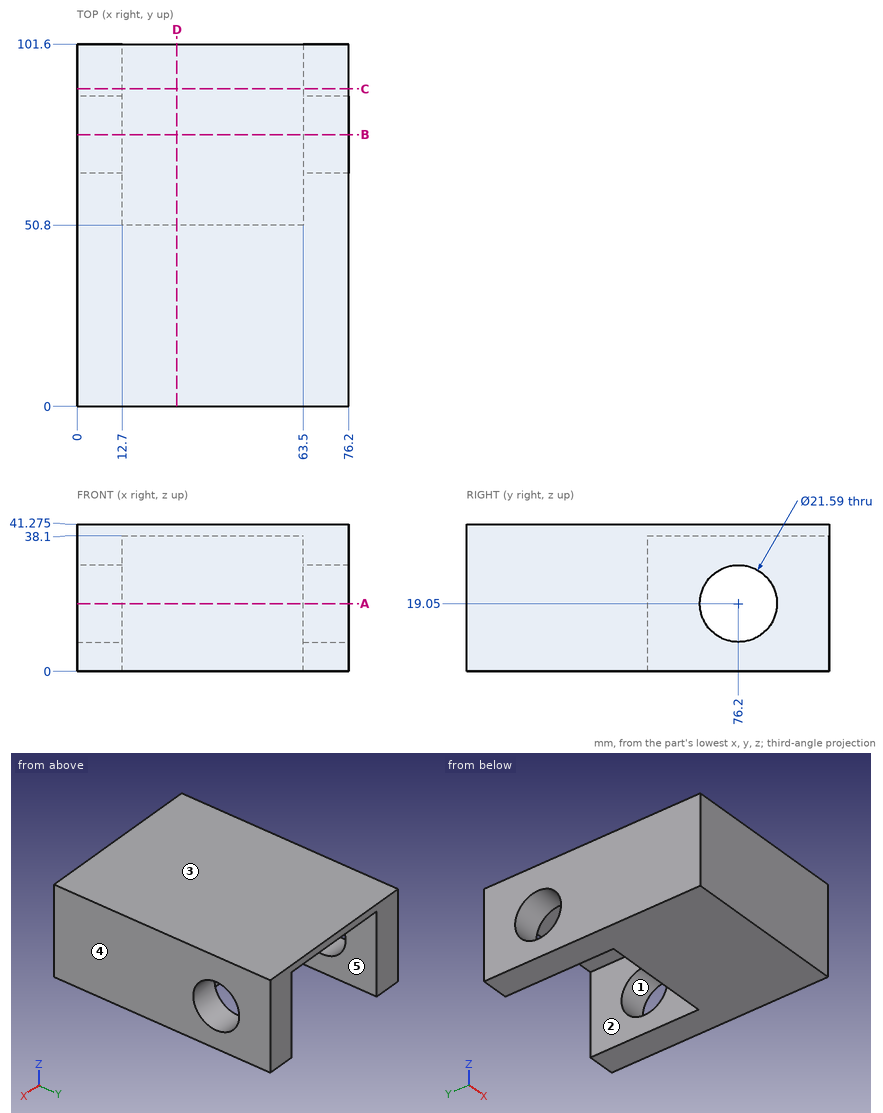
Answer from the drawing. Dimensions are ordinates in mm from the lowest x, y and z of the part. A direction names the side the tool comes from. Round coordinates to 2 decimals unless told otherwise and drop trailing zeros. Write each loop counter-clockwise with the first axis right and the second up, starting at its lowest first coordinate (ties: lowest second). Pieces come first, ordered by that corner, then holes. Notation, with made-up numbers: (19, 18.25) - (31, 18.25) arc R13 cw to (31, 35.25) - close; hole circle Ø3 at (-29.75, -27.75). An arc over 180 degrees is marked (long way). Use a Markdown table: item, result.
(1) The part is cut by section B-B (y = 76.2). Write down the section's boundary in (x, z) (3 decimals).
Reported:
| item | result |
|---|---|
| outline | (0, 0) - (12.7, 0) - (12.7, 8.255) - (0, 8.255) - close; (0, 29.845) - (12.7, 29.845) - (12.7, 38.1) - (63.5, 38.1) - (63.5, 29.845) - (76.2, 29.845) - (76.2, 41.275) - (0, 41.275) - close; (63.5, 0) - (76.2, 0) - (76.2, 8.255) - (63.5, 8.255) - close |
(2) The part is cut by section D-D (x = 28). Write down the section's boundary in (y, z) (3 decimals).
Reported:
| item | result |
|---|---|
| outline | (0, 0) - (50.8, 0) - (50.8, 38.1) - (101.6, 38.1) - (101.6, 41.275) - (0, 41.275) - close |
(3) This flat-tipped pin is pushed along its axis until it touches: pin 1 Ø1.5 at (x, z) = (47, 13.5) entering from +Y. Where does it stop, or does it pass through?
Reported:
| item | result |
|---|---|
| pin 1 | y = 50.8 |
(4) The part is cut by section C-C (y = 89). Write down the section's boundary in (x, z) (3 decimals), then the cut area to 3 significant figures.
Reported:
| item | result |
|---|---|
| outline | (0, 0) - (12.7, 0) - (12.7, 38.1) - (63.5, 38.1) - (63.5, 0) - (76.2, 0) - (76.2, 41.275) - (0, 41.275) - close |
| area | 1,210 mm2 |
(5) The part is cut by section A-A (z = 19.05). Write down the section's boundary in (x, y) (3 decimals).
Reported:
| item | result |
|---|---|
| outline | (0, 0) - (76.2, 0) - (76.2, 65.405) - (63.5, 65.405) - (63.5, 50.8) - (12.7, 50.8) - (12.7, 65.405) - (0, 65.405) - close; (0, 86.995) - (12.7, 86.995) - (12.7, 101.6) - (0, 101.6) - close; (63.5, 86.995) - (76.2, 86.995) - (76.2, 101.6) - (63.5, 101.6) - close |
(6) Which of the six approach directions +Z, -Z, +X, -X, +Y, -Y give full straight-line access (tool end or side, diameter ignored) to the marked faces 1 and 2?
Reported:
| item | result |
|---|---|
| face 1 | +X, -X |
| face 2 | -Z, +Y |
(7) Straight lines are drawn through the part: line 1 along Y through (x, z) = (72.5, 19.05) (3 decimals); line 2 along Z through (x, y) = (8, 76.2) (3 decimals); line 3 along X through (y, z) = (81, 33). For each, find the intervals that lie inside material, in ascending order. Write a range as [from, to].
Reported:
| item | result |
|---|---|
| line 1 | [0, 65.405], [86.995, 101.6] |
| line 2 | [0, 8.255], [29.845, 41.275] |
| line 3 | [0, 12.7], [63.5, 76.2] |
(8) The mould has two halves that part along X. Classify the marked faces 3, 4 and 5: released by +X, released by -X, zero draft, split by the parting line, or undercut.
Reported:
| item | result |
|---|---|
| face 3 | zero draft |
| face 4 | released by +X |
| face 5 | undercut |
